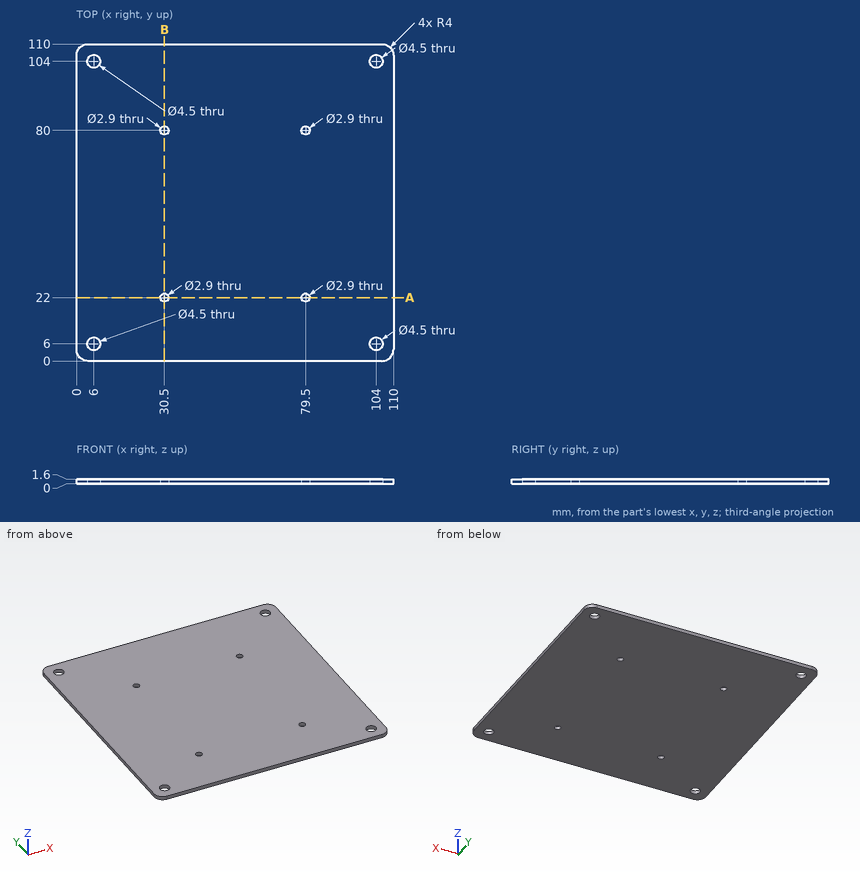
Check sheet for the drawn part. Datum: minimum x, y, z corner. Units: mm. Round coordinates to 2 decimals unless told otherwise and drop trailing zeros. Order: outer loops, then holes, each group sorted by start corner. A loop starts at its lowest first (then second) coordinate and runs counter-clockwise, first axis right, second up. Notation, with made-up numbers: (-10.5, 82.5) -> (23.5, 82.5) arc R17 cw to (23.5, 95.5) -> close; hole circle Ø11 at (81.5, -6). An arc over 180 degrees is marked (long way). Return JSON: item names as keys, results as strings. Group by question number.
Q1. Section check B-B, the plane x = 30.5. Record the boundary of the cut face in (y, z), plus the area to 3 significant figures.
Q2. Material ranges on probe 1 along X at (y, z) = (6, 0.9); probe 2 along X at (y, z) = (22, 1.2), recorded low to high. Write a range as from..to.
Q3. Section check A-A, the plane y = 22. Record the boundary of the cut face in (x, z).
Numbers:
{
 "1": {"outline": "(0, 0) -> (20.55, 0) -> (20.55, 1.6) -> (0, 1.6) -> close; (23.45, 0) -> (78.55, 0) -> (78.55, 1.6) -> (23.45, 1.6) -> close; (81.45, 0) -> (110, 0) -> (110, 1.6) -> (81.45, 1.6) -> close", "area": "167 mm^2"},
 "2": {"probe 1": "0..3.75, 8.25..101.75, 106.25..110", "probe 2": "0..29.05, 31.95..78.05, 80.95..110"},
 "3": {"outline": "(0, 0) -> (29.05, 0) -> (29.05, 1.6) -> (0, 1.6) -> close; (31.95, 0) -> (78.05, 0) -> (78.05, 1.6) -> (31.95, 1.6) -> close; (80.95, 0) -> (110, 0) -> (110, 1.6) -> (80.95, 1.6) -> close"}
}
